Source: three-view drawing plus pictorial views. Frame: mm from the lowest corner of the part. Round coordinates to 2 decimals unless told otherwise and drop trailing zeros. Order: outer loops, then holes, each group sorted by start corner. A loop starts at its lowest first (then second) coordinate and runs counter-clockwise, first axis right, second up. Notation, with made-up numbers: (-20.75, -15.75) -> (19.25, -15.75) arc R16 ccw to (19.25, 6.25) -> close; hole circle Ø10 at (-10, 36.25). An arc over 180 degrees is marked (long way). Use a Markdown table: item, result.
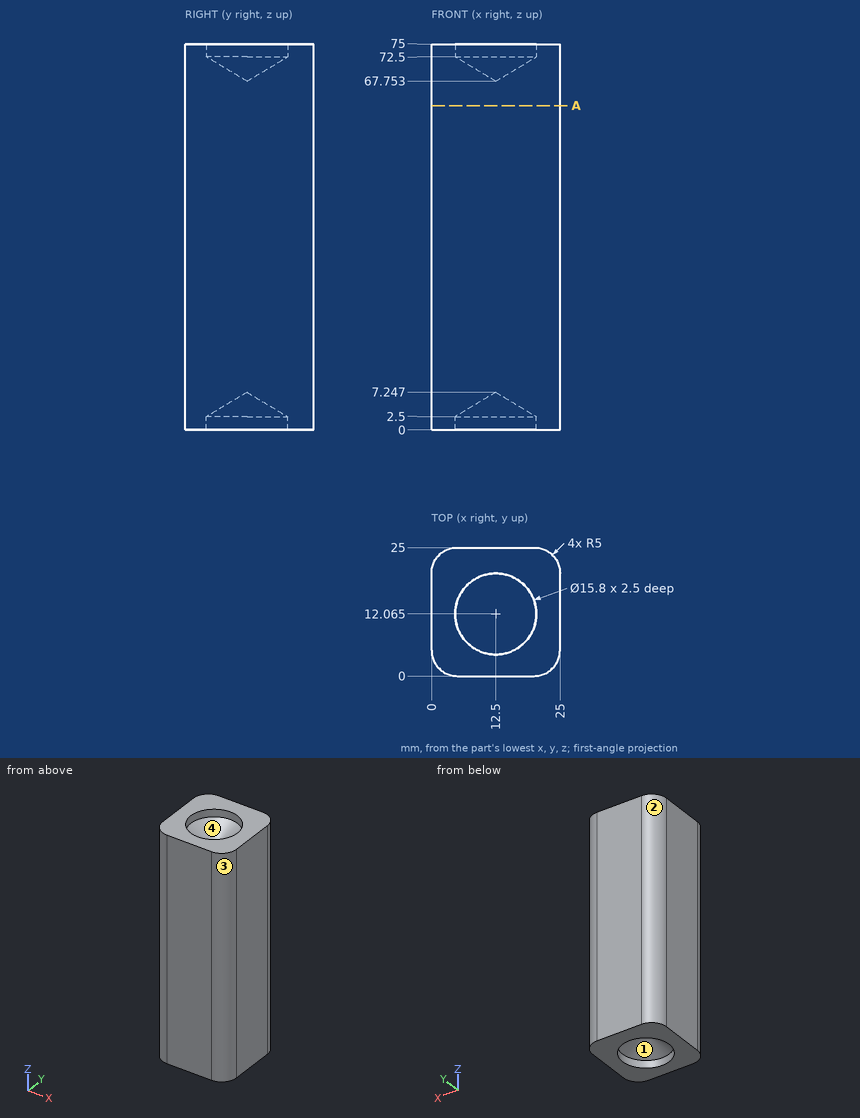
1) Pin query (flat end, axial travel): pin 1 Ø1.5 at (x, y) = (17, 11) entering from -Z; pin 2 Ø2 at (x, y) = (13.5, 12) entering from -Z (1 decimal); pin 3 Ø14 at (x, y) = (12.5, 12.06) entering from -Z. Return the tip coordinate at first contact, or that it passes through.
Results found:
| item | result |
|---|---|
| pin 1 | stops at z = 4.02 |
| pin 2 | stops at z = 6 |
| pin 3 | stops at z = 3.04 |
2) Line query: L1, parallel to Y at x = 12.5, z = 1.15 (1 decimal); L2, parallel to X at y = 12, z = 72 (1 decimal); L3, parallel to Z at x = 10.75, y = 12 (1 decimal). Output: solid intervals per line, ascending. Write a range as [from, to].
Results found:
| item | result |
|---|---|
| L1 | y = [0, 4.2], [20, 25] |
| L2 | x = [0, 5.4], [19.6, 25] |
| L3 | z = [6.2, 68.8] |
3) Cut plane A-A on z = 63. Return loops of the section in (x, y).
Results found:
| item | result |
|---|---|
| outline | (0, 5) arc R5 ccw to (5, 0) -> (20, 0) arc R5 ccw to (25, 5) -> (25, 20) arc R5 ccw to (20, 25) -> (5, 25) arc R5 ccw to (0, 20) -> close |
4) Pull-direction query (Y, two-part tool) for the marked faces 1, 2, 3 and 4; classes: +Y half, -Y half, draft (parallel to the pull), parting line (faces both ways), or undercut.
Results found:
| item | result |
|---|---|
| face 1 | undercut |
| face 2 | +Y half |
| face 3 | -Y half |
| face 4 | undercut |
